Check sheet for the drawn part. Datum: minimum x, y, z corner. Units: mm. A direction names the side the tool comes from. Round coordinates to 2 decimals unless told otherwise and drop trailing zeros. Loops run counter-clockwise (first coordinate to the right, second up) from the corner with the lowest first, then second, coordinate; pieces in that order, holes last.
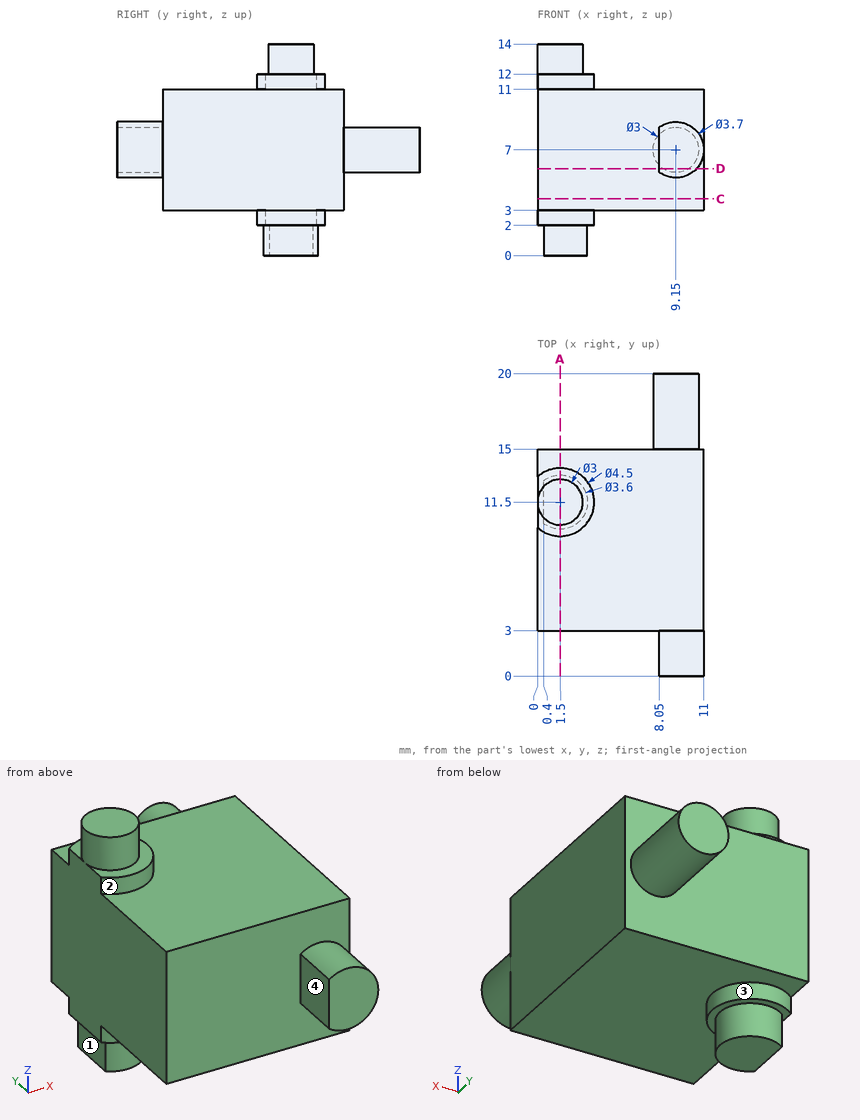
1) Access from +Z, -Z, +X, -X, +Y, -Y to the whole of each face (thin tool, end or side, straight path). Record for the marked faces 1, 2, 3 and 4.
Report:
face 1: -Z, -X, +Y, -Y
face 2: +Z
face 3: -Z
face 4: +Z, -Z, -X, -Y
2) Scan lines: line 1 along Z through (x, y) = (8.5, 7); line 2 along Y through (x, z) = (5.75, 5); line 3 along Y through (x, z) = (8, 6.5). Record each from-to range of solid material in increasing order.
Report:
line 1: z = 3 to 11
line 2: y = 3 to 15
line 3: y = 3 to 20
3) Gauge pin test, flat ends, axial feed: pin 1 (5.5 mm diameter, centred on x = 6, y = 7.5, fed in from -Z); pin 2 (0.6 mm diameter, centred on y = 12, z = 1, fed in from -X); pin 3 (1.5 mm diameter, centred on y = 17, z = 10.5, fed in from +X); pin 4 (5 mm diameter, centred on x = 1.5, z = 4.5, fed in from -Y). Record the tip position at first contact, or that the pin passes through.
Report:
pin 1: stops at z = 3
pin 2: stops at x = 0.4
pin 3: passes through
pin 4: stops at y = 3
4) Sectioned sample at A-A, the plane x = 1.5. Record the cut outline in (y, z).
Report:
outline: (3, 3) - (9.25, 3) - (9.25, 2) - (9.7, 2) - (9.7, 0) - (13.3, 0) - (13.3, 2) - (13.75, 2) - (13.75, 3) - (15, 3) - (15, 11) - (13.75, 11) - (13.75, 12) - (13, 12) - (13, 14) - (10, 14) - (10, 12) - (9.25, 12) - (9.25, 11) - (3, 11) - close
5) Sectioned sample at C-C, the plane z = 3.75. Record the cut outline in (x, y).
Report:
outline: (0, 3) - (11, 3) - (11, 15) - (0, 15) - close
6) Sectioned sample at D-D, the plane z = 5.75. Record the cut outline in (x, y), then the cut area to 3 significant figures.
Report:
outline: (0, 3) - (8.05, 3) - (8.05, 0) - (10.51, 0) - (10.51, 3) - (11, 3) - (11, 15) - (9.98, 15) - (9.98, 20) - (8.32, 20) - (8.32, 15) - (0, 15) - close
area: 148 mm2
